```python
from build123d import *

# Parameters (mm, degrees)
SKETCH1_W                      = 60
SKETCH1_H                      = 100
EXTRUDE1_DEPTH                 = 10
SKETCH2_W                      = 20
SKETCH2_H                      = 10
EXTRUDE2_DEPTH                 = 30.5
SKETCH4_W                      = 20
SKETCH4_H                      = 10
EXTRUDE3_DEPTH                 = 10
SKETCH5_R                      = 7.75
CUT_EXTRUDE1_DEPTH             = 3
SKETCH6_R                      = 4.8
CUT_EXTRUDE2_DEPTH             = 109.769738684
CBORE_FOR_M3_SHCS1_D           = 3.4
CBORE_FOR_M3_SHCS1_CBORE_D     = 6.5
CBORE_FOR_M3_SHCS1_CBORE_DEPTH = 3


with BuildPart() as part:
    # Sketch1 → Extrude1 (new body)
    with BuildSketch(Plane.XY):
        with Locations((-9.263291422, 28.303995668)):
            Rectangle(SKETCH1_W, SKETCH1_H)
    extrude(amount=EXTRUDE1_DEPTH)

    # Sketch2 → Extrude2 (add)
    with BuildSketch(Plane.XY.offset(10)):
        with Locations((-9.263291422, -16.696004332)):
            Rectangle(SKETCH2_W, SKETCH2_H)
    extrude(amount=EXTRUDE2_DEPTH)

    # Sketch4 → Extrude3 (add)
    with BuildSketch(Plane(origin=(0, -11.696004332, 0), x_dir=(1, 0, 0), z_dir=(0, 1, 0))):
        with Locations((-9.263291422, -35.5)):
            Rectangle(SKETCH4_W, SKETCH4_H)
    extrude(amount=EXTRUDE3_DEPTH)

    # Sketch5 → Cut-Extrude1 (cut)
    with BuildSketch(Plane(origin=(0, -11.696004332, 0), x_dir=(1, 0, 0), z_dir=(0, 1, 0))):
        with Locations(Location((-9.263291422, -20.25, 0), (0, 0, 270))):
            Circle(SKETCH5_R)
    extrude(amount=-CUT_EXTRUDE1_DEPTH, mode=Mode.SUBTRACT)

    # Sketch6 → Cut-Extrude2 (cut, through all)
    with BuildSketch(Plane(origin=(0, -14.696004332, 0), x_dir=(1, 0, 0), z_dir=(0, 1, 0))):
        with Locations(Location((-9.263291422, -20.25, 0), (0, 0, 270))):
            Circle(SKETCH6_R)
    extrude(amount=-CUT_EXTRUDE2_DEPTH, mode=Mode.SUBTRACT)

    # CBORE for M3 SHCS1 (through all)
    with Locations(Plane(origin=(-21.763291422, 68.303995668, 10), x_dir=(1, 0, 0), z_dir=(0, 0, 1))):
        with Locations((0, 0), (0, -25), (25, 0), (25, -25)):
            CounterBoreHole(CBORE_FOR_M3_SHCS1_D / 2, CBORE_FOR_M3_SHCS1_CBORE_D / 2, CBORE_FOR_M3_SHCS1_CBORE_DEPTH)


solid = part.part
```
Can you work these out from the model? Positions are in its coordinate system, mm. A direction names the side the tool comes from. Give positions to 0.01 mm unless a question says otherwise; leave off trailing zeros. Loops run counter-clockwise (first coordinate to the right, second up) from the corner with the lowest first, then second, coordinate; pieces in that order, holes last. Notation, with made-up numbers: M 65.5,81.5 L 88.5,81.5 A12 ccw 88.5,103.5 Z; hole C 50,-38 d7. An arc over 180 degrees is marked long. Answer in a Markdown table with one row per item.
1. Which directions (+Z, -Z, +X, -X, +Y, -Y) give clear straight access to the entire face, cutting with the end or side of a thin tool? Please do faces 4 (the flat face through (5, 42, 7)), 5 (the cylindrical face through (-22.548, 41.796, 3.451)), 6 (the flat face through (-16, -11.696, 16)), 7 (the flat face through (-19.263, -14, 29)).
Taken from the geometry:
| item | result |
|---|---|
| face 4 | +Z |
| face 5 | +Z, -Z |
| face 6 | +X, -X, +Y |
| face 7 | +Z, -X, +Y, -Y |
2. Suppose I cut it at C-C on y = 23. Write out the boundary of the cut face in (x, z).
Taken from the geometry:
| item | result |
|---|---|
| outline | M -39.26,0 L 20.74,0 L 20.74,10 L -39.26,10 Z |
3. Thinking about a two-plate mould opening in Y: for faces 1 (the flat face through (0.737, -14, 29)), 2 (the flat face through (-6, -14.696, 24)), 3 (the cylindrical face through (-22.186, 71.526, 8.521)), which applies, released by +Y, released by -Y, zero draft, split by the parting line, or undercut?
Taken from the geometry:
| item | result |
|---|---|
| face 1 | zero draft |
| face 2 | released by +Y |
| face 3 | undercut |
4. If I drill on line 1 along X through (y, z) = (-19.5, 20.25); line 2 along X through (y, z) = (-13, 20); line 3 along Y through (x, z) = (-4, 34), over which ranges is the centre line in solid material (lowest first)?
Taken from the geometry:
| item | result |
|---|---|
| line 1 | x = -19.26 to -14.06, -4.46 to 0.74 |
| line 2 | x = -19.26 to -17.01, -1.52 to 0.74 |
| line 3 | y = -21.7 to -1.7 |
5. Suppose I cut it at D-D on z = 38.5. Write out the boundary of the cut face in (x, y), plus the area to 3 significant figures.
Taken from the geometry:
| item | result |
|---|---|
| outline | M -19.26,-21.7 L 0.74,-21.7 L 0.74,-1.7 L -19.26,-1.7 Z |
| area | 400 mm² |
6. Suppose I cut it at A-A on z = 20.25. Write out the boundary of the cut face in (x, y).
Taken from the geometry:
| item | result |
|---|---|
| outline | M -19.26,-21.7 L -14.06,-21.7 L -14.06,-14.7 L -17.01,-14.7 L -17.01,-11.7 L -19.26,-11.7 Z; M -4.46,-21.7 L 0.74,-21.7 L 0.74,-11.7 L -1.51,-11.7 L -1.51,-14.7 L -4.46,-14.7 Z |
7. Suppose I cut it at B-B on x = -22. Write out the boundary of the cut face in (y, z), plus the area to 3 significant figures.
Taken from the geometry:
| item | result |
|---|---|
| outline | M -21.7,0 L 41.62,0 L 41.62,7 L 40.06,7 L 40.06,10 L -21.7,10 Z; M 44.99,0 L 66.62,0 L 66.62,7 L 65.06,7 L 65.06,10 L 46.55,10 L 46.55,7 L 44.99,7 Z; M 69.99,0 L 78.3,0 L 78.3,10 L 71.55,10 L 71.55,7 L 69.99,7 Z |
| area | 914 mm² |
8. For pin 1 Ø10 at (y, z) = (-13.5, 24.5) entering from +X; pin 2 Ø12 at (x, y) = (12, 51) entering from +Z; pin 3 Ø8 at (x, z) = (-11, 23) entering from +Y, each with a flat end and sliding along its axis, tell me the tip position at first contact or that it passes through.
Taken from the geometry:
| item | result |
|---|---|
| pin 1 | stops at x = 0.74 |
| pin 2 | stops at z = 10 |
| pin 3 | stops at y = -14.7 |
